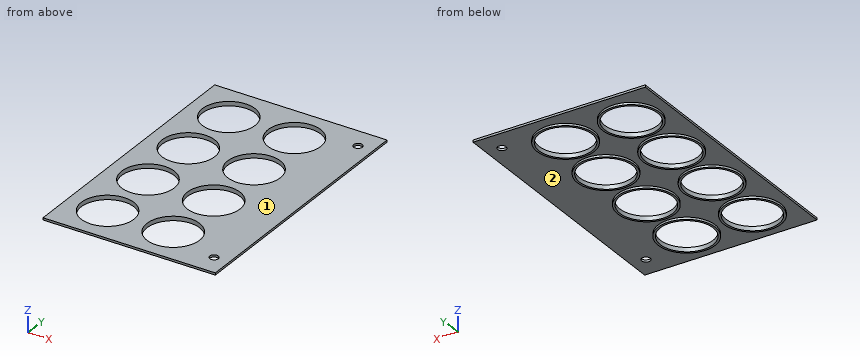
from build123d import *

# Parameters (mm, degrees)
F0_W     = 80
F0_H     = 124
F0_R     = 13.25
F0_R_2   = 12.25
F4_R     = 2
F5_DEPTH = 2


with BuildPart() as f2:
    # F2: sweep along a path in F1
    with BuildLine(Plane.YZ) as f2_path:
        Line((62, 0), (62, -1))
    # F0 (on Top) → F2 (sweep)
    with BuildSketch(Plane.XY):
        Rectangle(F0_W, F0_H)
        with Locations((-21.75, -43.75)):
            Circle(F0_R, mode=Mode.SUBTRACT)
        with Locations((-21.75, -14.583333)):
            Circle(F0_R, mode=Mode.SUBTRACT)
        with Locations((8.75, -43.75)):
            Circle(F0_R, mode=Mode.SUBTRACT)
        with Locations((8.75, -14.583333)):
            Circle(F0_R, mode=Mode.SUBTRACT)
        with Locations((-21.75, 14.583333)):
            Circle(F0_R, mode=Mode.SUBTRACT)
        with Locations((-21.75, 43.75)):
            Circle(F0_R, mode=Mode.SUBTRACT)
        with Locations((8.75, 14.583333)):
            Circle(F0_R, mode=Mode.SUBTRACT)
        with Locations((8.75, 43.75)):
            Circle(F0_R, mode=Mode.SUBTRACT)
    sweep(path=f2_path.line)

    # F3: sweep along a path in F1
    with BuildLine(Plane.YZ) as f3_path:
        Line((62, 0), (62, -1))
        Line((62, -1), (62, -2))
    # F0 (on Top) → F3 (sweep)
    with BuildSketch(Plane.XY):
        with Locations((-21.75, -14.583333)):
            Circle(F0_R)
        with Locations((-21.75, -14.583333)):
            Circle(F0_R_2, mode=Mode.SUBTRACT)
        with Locations((-21.75, 14.583333)):
            Circle(F0_R)
        with Locations((-21.75, 14.583333)):
            Circle(F0_R_2, mode=Mode.SUBTRACT)
        with Locations((-21.75, -43.75)):
            Circle(F0_R)
        with Locations((-21.75, -43.75)):
            Circle(F0_R_2, mode=Mode.SUBTRACT)
        with Locations((8.75, -43.75)):
            Circle(F0_R)
        with Locations((8.75, -43.75)):
            Circle(F0_R_2, mode=Mode.SUBTRACT)
        with Locations((8.75, -14.583333)):
            Circle(F0_R)
        with Locations((8.75, -14.583333)):
            Circle(F0_R_2, mode=Mode.SUBTRACT)
        with Locations((8.75, 14.583333)):
            Circle(F0_R)
        with Locations((8.75, 14.583333)):
            Circle(F0_R_2, mode=Mode.SUBTRACT)
        with Locations((8.75, 43.75)):
            Circle(F0_R)
        with Locations((8.75, 43.75)):
            Circle(F0_R_2, mode=Mode.SUBTRACT)
        with Locations((-21.75, 43.75)):
            Circle(F0_R)
        with Locations((-21.75, 43.75)):
            Circle(F0_R_2, mode=Mode.SUBTRACT)
    sweep(path=f3_path.line)

    # F4 (on face) → F5 (cut)
    with BuildSketch(Plane.XY):
        with Locations((33, 52)):
            Circle(F4_R)
        with Locations((33, -52)):
            Circle(F4_R)
    extrude(amount=-F5_DEPTH, mode=Mode.SUBTRACT)


solid = f2.part
Build history of the part. All positions in model axes, mm. Face numbers are marked on the shaded views. Give positions to 0.01 mm unless a question says otherwise; leave off trailing zeros. Write each loop counter-clockwise with the first axis right and the second up, starting at its lowest first coordinate (ties: lowest second). Pieces come first, ordered by that corner, then holes. Notation, with made-up numbers: (73, -5) - (110, -5) arc R27 cw to (110, 22) - close; hole circle Ø7 at (26.5, 6.25). An arc over 180 degrees is marked (long way). Use one line per item in the form item = value. Start each with the question number.
1. Band-saw the part on B-B on x = 33. Write the cut outline in (y, z), plus the area to 3 significant figures.
2. Band-saw the part on D-D on y = -8. Write the cut outline in (x, z), plus the area to 4 significant figures.
3. Two-plate mould, pull along Y, no slides. Class the marked faces 1 and 2: released by +Y, released by -Y, zero draft, split by the parting line, or undercut.
4. Band-saw the part on A-A on y = 43.75. Write the cut outline in (x, z).
5. Band-saw the part on C-C on z = -1.6. Count the separate pieces of the cut face and the enclosed holes in it, plus the area to 3 significant figures.
6. Drop flat-ended pins along their axis: pin 1 Ø6 at (x, y) = (14.5, 47.5) entering from +Z; pin 2 Ø1 at (x, z) = (16, -2) entering from +Y. Give the stop position or say it passes through.
7. Probe line 1 (Y direction, x = 8.75, z = -0.75); line 2 (Y direction, x = 33, z = -0.2); line 3 (X direction, y = -7, z = -1.15). List the from-to ranges inside material, lowest first. Write a range as [from, to].
Conclusion:
q1.outline = (-62, -1) - (-54, -1) - (-54, 0) - (-62, 0) - close; (-50, -1) - (50, -1) - (50, 0) - (-50, 0) - close; (54, -1) - (62, -1) - (62, 0) - (54, 0) - close
q1.area = 116 mm²
q2.outline = (-40, -1) - (-33.25, -1) - (-33.25, -2) - (-32.08, -2) - (-32.08, 0) - (-40, 0) - close; (-11.42, -2) - (-10.25, -2) - (-10.25, -1) - (-2.75, -1) - (-2.75, -2) - (-1.58, -2) - (-1.58, 0) - (-11.42, 0) - close; (19.08, -2) - (20.25, -2) - (20.25, -1) - (40, -1) - (40, 0) - (19.08, 0) - close
q2.area = 43.35 mm²
q3.face_1 = zero draft
q3.face_2 = undercut
q4.outline = (-40, -1) - (-35, -1) - (-35, -2) - (-34, -2) - (-34, 0) - (-40, 0) - close; (-9.5, -2) - (-8.5, -2) - (-8.5, -1) - (-4.5, -1) - (-4.5, -2) - (-3.5, -2) - (-3.5, 0) - (-9.5, 0) - close; (21, -2) - (22, -2) - (22, -1) - (40, -1) - (40, 0) - (21, 0) - close
q5.separate_pieces = 8
q5.enclosed_holes = 8
q5.area = 641 mm²
q6.pin_1 = through
q6.pin_2 = 55.15
q7.line_1 = [-62, -56], [-31.5, -26.83], [-2.33, 2.33], [26.83, 31.5], [56, 62]
q7.line_2 = [-62, -54], [-50, 50], [54, 62]
q7.line_3 = [-32.62, -31.37], [-12.13, -10.88], [-2.12, -0.87], [18.37, 19.62]
